from build123d import *

# Parameters (mm, degrees)
SKETCH1_W           = 25.4
SKETCH1_H           = 50.8
SKETCH1_W_2         = 20.32
SKETCH1_H_2         = 45.72
EXTRUDE_THIN1_DEPTH = 46.0375
SKETCH2_R           = 2.4765
CUT_EXTRUDE1_DEPTH  = 51.8


with BuildPart() as part:
    # Sketch1 → Extrude-Thin1 (new body, symmetric)
    with BuildSketch(Plane.XY):
        Rectangle(SKETCH1_W, SKETCH1_H)
        Rectangle(SKETCH1_W_2, SKETCH1_H_2, mode=Mode.SUBTRACT)
    extrude(amount=EXTRUDE_THIN1_DEPTH, both=True)

    # Sketch2 → Cut-Extrude1 (cut, through all)
    with BuildSketch(Plane.XZ.offset(25.4)):
        with Locations((-5.11e-06, 33.3375)):
            Circle(SKETCH2_R)
    extrude(amount=-CUT_EXTRUDE1_DEPTH, mode=Mode.SUBTRACT)


solid = part.part
CAD build for the part. Positions are in the model's coordinates, mm. A direction names the side the tool comes from. Round coordinates to 2 decimals unless told otherwise and drop trailing zeros. Order: outer loops, then holes, each group sorted by start corner. A loop starts at its lowest first (then second) coordinate and runs counter-clockwise, first axis right, second up. Notation, with made-up numbers: (-1, 28) -> (10, 28) arc R22 ccw to (10, 59) -> close; hole circle Ø2 at (76, 25.5). An arc over 180 degrees is marked (long way). Write item = value, one per line. Start each with the question number.
(1) Pull direction X, two halves, no side cores. Call faces 1 (the flat face through (-12.7, 0, 1)), 2 (the flat face through (0, 22.86, 1)), 3 (the flat face through (12.7, 0, 1)), 4 (the flat face through (0, 25.4, 1)): released by +X, released by -X, zero draft, split by the parting line, or undercut.
(2) Cut at B-B, the plane x = 0. List the corners of the cut face in (y, z).
(3) Cut at C-C, the plane y = 4. List the corners of the cut face in (x, z).
(4) Which spindle directions (+Z, -Z, +X, -X, +Y, -Y) get a long thin tool onto all of the face, cutting with end or side? Do faces 5 (the flat face through (0, -22.86, 1)), 6 (the cylindrical face through (-0.54, 24.11, 30.92)). Say none if no direction does.
(5) Cut at D-D, the plane x = 6.25. List the corners of the cut face in (y, z).
(6) Cut at A-A, the plane z = -18. List the corners of the cut face in (x, y), then the cut area to 3 significant figures.
(7) Probe line 1 (X direction, y = 20, z = 27); line 2 (Y direction, x = 0.75, z = 11). List the from-to ranges inside material, lowest first. Write a range as [from, to].
(8) Pin check, flat tips, straight feed: P1, Ø6.5, axis at x = 0, z = 33.34, coming from the +Y side; P2, Ø3, axis at x = -8, y = 14.5, coming from the -Z side. Stop position of each tip, or through.
Model answer:
q1.face_1 = released by -X
q1.face_2 = undercut
q1.face_3 = released by +X
q1.face_4 = zero draft
q2.outline = (-25.4, -46.04) -> (-22.86, -46.04) -> (-22.86, 30.86) -> (-25.4, 30.86) -> close; (-25.4, 35.81) -> (-22.86, 35.81) -> (-22.86, 46.04) -> (-25.4, 46.04) -> close; (22.86, -46.04) -> (25.4, -46.04) -> (25.4, 30.86) -> (22.86, 30.86) -> close; (22.86, 35.81) -> (25.4, 35.81) -> (25.4, 46.04) -> (22.86, 46.04) -> close
q3.outline = (-12.7, -46.04) -> (-10.16, -46.04) -> (-10.16, 46.04) -> (-12.7, 46.04) -> close; (10.16, -46.04) -> (12.7, -46.04) -> (12.7, 46.04) -> (10.16, 46.04) -> close
q4.face_5 = +Z, -Z
q4.face_6 = +Y, -Y
q5.outline = (-25.4, -46.04) -> (-22.86, -46.04) -> (-22.86, 46.04) -> (-25.4, 46.04) -> close; (22.86, -46.04) -> (25.4, -46.04) -> (25.4, 46.04) -> (22.86, 46.04) -> close
q6.outline = (-12.7, -25.4) -> (12.7, -25.4) -> (12.7, 25.4) -> (-12.7, 25.4) -> close; hole (-10.16, -22.86) -> (10.16, -22.86) -> (10.16, 22.86) -> (-10.16, 22.86) -> close
q6.area = 361 mm2
q7.line_1 = [-12.7, -10.16], [10.16, 12.7]
q7.line_2 = [-25.4, -22.86], [22.86, 25.4]
q8.P1 = 25.4
q8.P2 = through
